CAD build for the part. Positions are in the model's coordinates, mm. Give positions to 0.01 mm unless a question says otherwise; leave off trailing zeros. Loops run counter-clockwise (first coordinate to the right, second up) from the corner with the lowest first, then second, coordinate; pieces in that order, holes last.
Item 1: Saw through at A-A on x = 0. Give the cut face in (y, z).
Item 2: Saw through at B-B on x = 12. Give the number of separate pieces and of enclosed holes in the cut face, plus the area to 3 significant figures.
Item 3: Mould opens along X. For faces 1 (the cylindrical face through (-12.277, -21.359, -55.288)), 2 (the flat face through (-1, -43.18, 1)), 3 (the cylindrical face through (0.068, -21.288, -39.465)) say: released by +X, released by -X, zero draft, split by the parting line, or undercut.
Item 4: Drop flat-ended pins along their axis: P1, Ø12, axis at x = 43, y = -11, coming from the -Z side; P2, Ø1, axis at x = 38, y = -27, coming from the -Z side; P3, Ø12, axis at y = -38, z = -20, coming from the -X side; P4, Ø3, axis at y = -38, z = 1.5, coming from the -X side. Give the stop position or say it passes through.
Item 5: Probe probe 1 along X at (y, z) = (-23, 25); probe 2 along X at (y, z) = (-35.5, 19.5); probe 3 along Z at (x, y) = (-25, -23). List the from-to ranges inside material, lowest first.
from build123d import *

# Parameters (mm, degrees)
F0_R     = 56.634514
F0_R_2   = 14.25202
F1_DEPTH = 43.18
F2_R     = 5.08


with BuildPart() as f1:
    # F0 (on Front) → F1 (new body)
    with BuildSketch(Plane.XZ):
        Circle(F0_R)
        with BuildLine():
            ThreePointArc((36.836641, -14.160916), (-0.605346, -39.460147), (-37.253682, -13.024319))
            Line((-37.253682, -13.024319), (36.836641, -14.160916))
        make_face(mode=Mode.SUBTRACT)
        with Locations((-24.897231, 17.987859)):
            Circle(F0_R_2, mode=Mode.SUBTRACT)
        with Locations((24.897231, 17.987859)):
            Circle(F0_R_2, mode=Mode.SUBTRACT)
    extrude(amount=F1_DEPTH)

    # F2
    f2_edges = [f1.edges().sort_by_distance(p)[0] for p in [
        (-56.634514, -43.18, 0),
        (56.634514, -21.59, 0),
        (-56.634514, 0, 0),
    ]]
    fillet(f2_edges, radius=F2_R)


solid = f1.part
Results below:
1. outline: (-43.18, -51.55) arc R5.08 ccw to (-38.1, -56.63) - (-5.08, -56.63) arc R5.08 ccw to (0, -51.55) - (0, -39.46) - (-43.18, -39.46) - close; (-43.18, -13.6) - (0, -13.6) - (0, 51.55) arc R5.08 ccw to (-5.08, 56.63) - (-38.1, 56.63) arc R5.08 ccw to (-43.18, 51.55) - close
2. separate pieces: 3
2. enclosed holes: 0
2. area: 3,210 mm2
3. face 1: split by the parting line
3. face 2: zero draft
3. face 3: undercut
4. P1: stops at z = -42.88
4. P2: stops at z = -42.44
4. P3: stops at x = -54.88
4. P4: stops at x = -56.63
5. probe 1: x = -50.82 to -37.3, -12.49 to 12.49, 37.3 to 50.82
5. probe 2: x = -53.17 to -39.07, -10.73 to 10.73, 39.07 to 53.17
5. probe 3: z = -50.82 to -30.54, -13.21 to 3.74, 32.24 to 50.82
